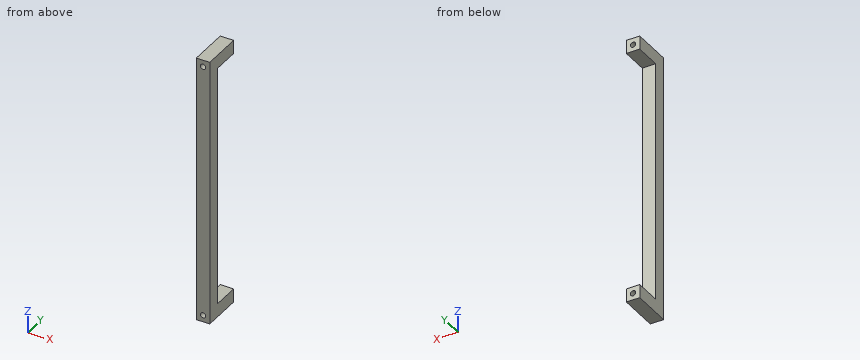
Autodesk Inventor part; units mm, degrees
ref_plane "YZ Plane" through (0, 0, 0) normal (1, 0, 0) x (0, 1, 0)
ref_plane "XZ Plane" through (0, 0, 0) normal (0, 1, 0) x (-1, 0, 0)
ref_plane "XY Plane" through (0, 0, 0) normal (0, 0, 1) x (1, 0, 0)
sketch "Sketch1" plane through (0, 0, 0) normal (0, 1, 0) x (-1, 0, 0)
  line L0 (0, 0) -> (-12.7, 0)
  line L1 (-12.7, 0) -> (-12.7, -254)
  line L2 (-12.7, -254) -> (0, -254)
  line L3 (0, -254) -> (0, 0)
  dimension "d0" = 254
  dimension "d1" = 12.7
extrude "Extrusion1" add sketch "Sketch1" along normal blind 12.7
sketch "Sketch2" plane through (0, 12.7, 0) normal (0, 1, 0) x (1, 0, 0)
  line L0 (12.7, 0) -> (12.7, 254)
  line L1 (0, 0) -> (12.7, 0)
  line L2 (12.7, 0) -> (12.7, 12.7)
  line L3 (12.7, 12.7) -> (0, 12.7)
  line L4 (0, 12.7) -> (0, 0)
  line L5 (12.7, 254) -> (0, 254)
  line L6 (0, 254) -> (12.7, 254)
  line L7 (12.7, 254) -> (12.7, 241.3)
  line L8 (12.7, 241.3) -> (0, 241.3)
  line L9 (0, 241.3) -> (0, 254)
  dimension "d4" = 12.7
extrude "Extrusion2" add sketch "Sketch2" along normal blind 25.4
sketch "Sketch3" plane through (0, 38.1, 0) normal (0, 1, 0) x (1, 0, 0)
  circle A0 centre (6.35, 6.35) radius 2.5019
  line L0 (0, 0) -> (12.7, 0)
  line L1 (12.7, 0) -> (12.7, 12.7)
  circle A1 centre (6.35, 247.65) radius 2.5019
  dimension "d7" = 5.0038
  dimension "d8" = 6.35
  dimension "d9" = 6.35
  dimension "d12" = 241.3
extrude "Extrusion3" cut sketch "Sketch3" against normal up to surface (38.1 mm away)
properties part number "handle ds"
The listing builds one solid part. Answer for the finished solid, in the listing's coordinates (mm). Round coordinates to 2 decimals unless told otherwise and drop trailing zeros. Write each loop counter-clockwise with the first axis right and the second up, starting at its lowest first coordinate (ties: lowest second). Pieces come first, ordered by that corner, then holes. Notation, with made-up numbers: M 75,-33.75 L 92,-33.75 A13 cw 92,-17.75 Z; hole C 40.5,23 d11. An arc over 180 degrees is marked long. Write each question's results on one line, items separated by ' | '. Start each with the question number.
(1) The part is cut by section B-B, the plane z = -6.35. Write down the section's boundary in (x, y).
(2) The part is cut by section D-D, the plane z = -126. Write down the section's boundary in (x, y).
(3) The part is cut by section C-C, the plane x = 6.35. Write down the section's boundary in (y, z), and give its area (3 significant figures).
(4) The part is cut by section A-A, the plane y = 15. Write down the section's boundary in (x, z), and give its area (3 significant figures).
(5) Find the intervals of material crossed by line 1 (Z direction, x = 6.35, y = 15); line 2 (Z direction, x = 10, y = 19.5); line 3 (Z direction, x = 8.5, y = 33), in increasing order.
(6) Each of these flat-tipped pins is pushed along its axis until it touches: P1, Ø4, axis at x = 6.35, z = -6.35, coming from the +Y side; P2, Ø2, axis at x = 4.5, y = 16.5, coming from the +Z side. Where does it stop, or does it pass through?
Worked answers:
1) outline: M 0,0 L 3.85,0 L 3.85,38.1 L 0,38.1 Z; M 8.85,0 L 12.7,0 L 12.7,38.1 L 8.85,38.1 Z
2) outline: M 0,0 L 12.7,0 L 12.7,12.7 L 0,12.7 Z
3) outline: M 0,-254 L 38.1,-254 L 38.1,-250.15 L 0,-250.15 Z; M 0,-245.15 L 38.1,-245.15 L 38.1,-241.3 L 12.7,-241.3 L 12.7,-12.7 L 38.1,-12.7 L 38.1,-8.85 L 0,-8.85 Z; M 0,-3.85 L 38.1,-3.85 L 38.1,0 L 0,0 Z | area: 3,490 mm²
4) outline: M 0,-254 L 12.7,-254 L 12.7,-241.3 L 0,-241.3 Z; M 0,-12.7 L 12.7,-12.7 L 12.7,0 L 0,0 Z; hole C 6.35,-247.65 d5; hole C 6.35,-6.35 d5 | area: 283 mm²
5) line 1: z = -254 to -250.15, -245.15 to -241.3, -12.7 to -8.85, -3.85 to 0 | line 2: z = -254 to -241.3, -12.7 to 0 | line 3: z = -254 to -248.93, -246.37 to -241.3, -12.7 to -7.63, -5.07 to 0
6) P1: passes through | P2: stops at z = 0
